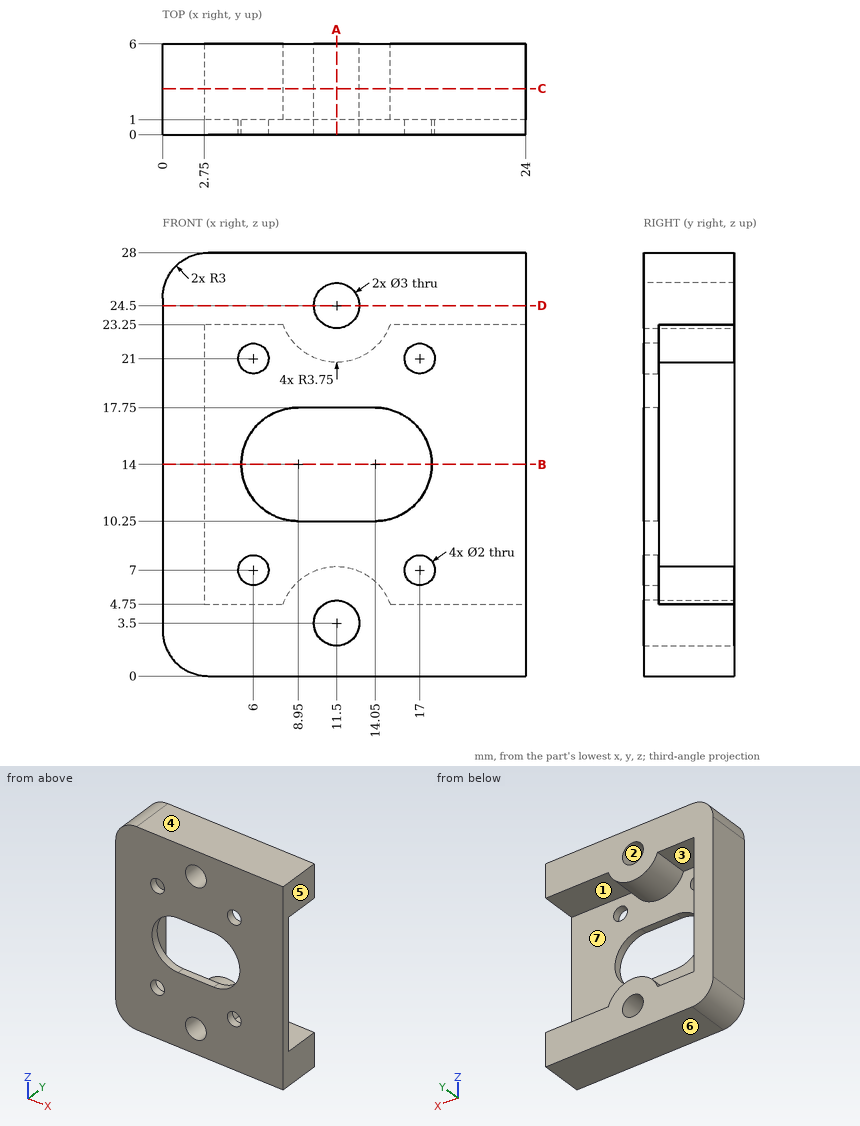
Check sheet for the drawn part. Datum: minimum x, y, z corner. Units: mm. A direction names the side the tool comes from. Round coordinates to 2 decimals unless told otherwise and drop trailing zeros. Loops run counter-clockwise (first coordinate to the right, second up) from the corner with the lowest first, then second, coordinate; pieces in that order, holes last. Notation, with made-up numbers: (84, 57) - (110, 57) arc R24 cw to (110, 73) - close; hole circle Ø9 at (-24, 14). An arc over 180 degrees is marked (long way). Write each question's results on one line, items separated by ' | '. Start each with the question number.
Q1. Release check for a two-part mould opening along Z. For the marked faces 4, 5, 6 and 7 record: +Z half, -Z half, draft (parallel to the pull), parting line (faces both ways), or undercut.
Q2. Cross-section at D-D on z = 24.5. Enter the section's corners in (x, y), and give its area (3 significant figures).
Q3. Cross-section at A-A on x = 11.5. Enter the section's corners in (y, z).
Q4. Gauge pin test, flat ends, axial feed: P1, Ø3, axis at x = 15, z = 9, coming from the +Y side; P2, Ø1.5, axis at y = 4.5, z = 11.5, coming from the +X side; P3, Ø1.8, axis at x = 17, z = 7, coming from the -Y side. Record the tip position at first contact, or that the pin passes through.
Q5. Cross-section at C-C on y = 3.05. Enter the section's corners in (x, z).
Q6. Cross-section at B-B on z = 14. Enter the section's corners in (x, y).
Q7. Thickness scan on line 1 (X direction, y = 0.85, z = 7); line 2 (X direction, y = 2.1, z = 24.5); line 3 (Z direction, x = 23.25, y = 2.75). Record the ranges inside material, lowest first. Write a range as [from, to].
Q8. Access from +Z, -Z, +X, -X, +Y, -Y to the whole of each face (thin tool, end or side, straight path). Record for the marked faces 1, 2 and 3.
Answers below:
1) face 4: +Z half | face 5: draft | face 6: -Z half | face 7: undercut
2) outline: (0, 0) - (10, 0) - (10, 6) - (0, 6) - close; (13, 0) - (24, 0) - (24, 6) - (13, 6) - close | area: 126 mm²
3) outline: (0, 0) - (6, 0) - (6, 2) - (0, 2) - close; (0, 5) - (6, 5) - (6, 7.25) - (1, 7.25) - (1, 10.25) - (0, 10.25) - close; (0, 17.75) - (1, 17.75) - (1, 20.75) - (6, 20.75) - (6, 23) - (0, 23) - close; (0, 26) - (6, 26) - (6, 28) - (0, 28) - close
4) P1: stops at y = 1 | P2: stops at x = 2.75 | P3: passes through
5) outline: (0, 3) arc R3 ccw to (3, 0) - (24, 0) - (24, 4.75) - (15.04, 4.75) arc R3.75 ccw to (7.96, 4.75) - (2.75, 4.75) - (2.75, 23.25) - (7.96, 23.25) arc R3.75 ccw to (15.04, 23.25) - (24, 23.25) - (24, 28) - (3, 28) arc R3 ccw to (0, 25) - close; hole circle Ø3 at (11.5, 3.5); hole circle Ø3 at (11.5, 24.5)
6) outline: (0, 0) - (5.2, 0) - (5.2, 1) - (2.75, 1) - (2.75, 6) - (0, 6) - close; (17.8, 0) - (24, 0) - (24, 1) - (17.8, 1) - close
7) line 1: x = [0, 5], [7, 16], [18, 24] | line 2: x = [0, 10], [13, 24] | line 3: z = [0, 4.75], [23.25, 28]
8) face 1: +X, +Y | face 2: +Y, -Y | face 3: +Y
